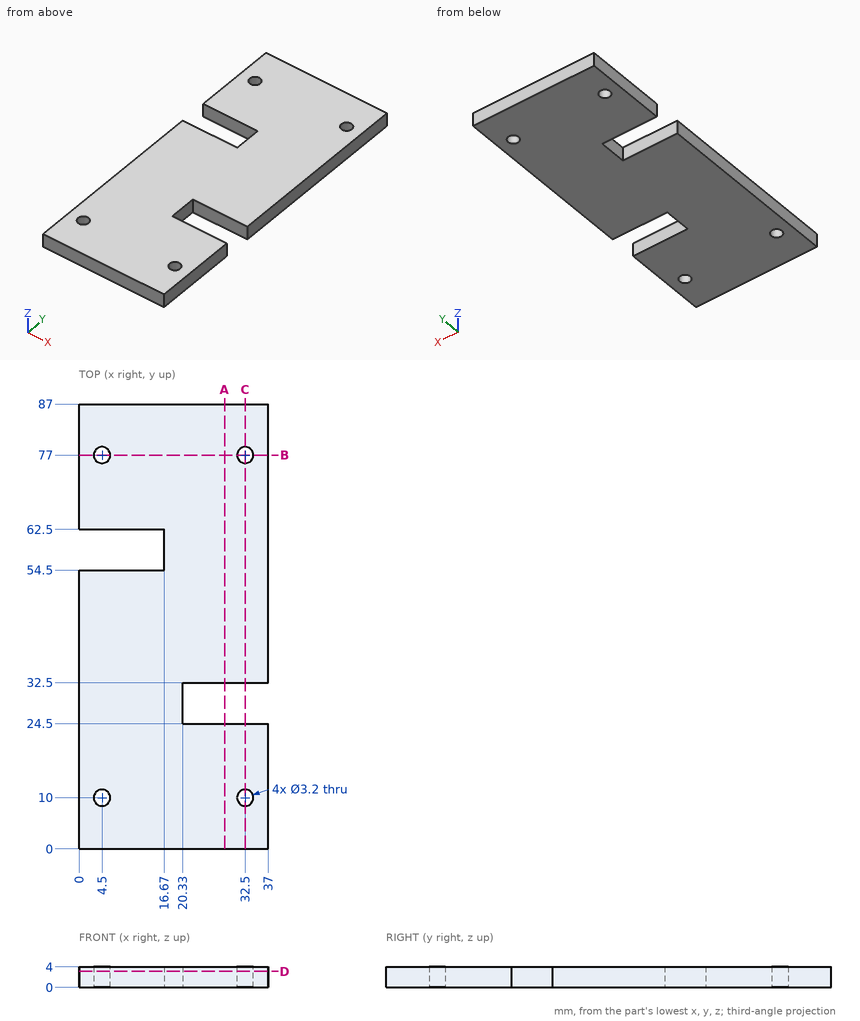
Geometry check sheet. Reference: drawing and pictorial views, mm from the part's lowest x, y, z. Give positions to 0.01 mm unless a question says otherwise; leave off trailing zeros. Order: outer loops, then holes, each group sorted by start corner. A loop starts at its lowest first (then second) coordinate and runs counter-clockwise, first axis right, second up. Notation, with made-up numbers: (58.5, -36) -> (87.5, -36) arc R31 cw to (87.5, -3) -> close; hole circle Ø4 at (22.5, 9). An arc over 180 degrees is marked (long way). Use CSV: the item, a comma, the result in double quotes. Start each with the question number.
1) Sectioned sample at D-D, the plane z = 3.1. Record the boundary of the cut face in (x, y).
2) Sectioned sample at A-A, the plane x = 28.5. Record the boundary of the cut face in (y, z).
3) Go/stop test with a flat-tipped pin: P1, Ø5, axis at x = 4.5, y = 77, coming from the -Z side. Record where the tip stops, or that it passes through.
4) Sectioned sample at B-B, the plane y = 77. Record the boundary of the cut face in (x, z), plus the area to 3 significant figures.
5) Sectioned sample at C-C, the plane x = 32.5. Record the boundary of the cut face in (y, z).
6) Material ranges on line 1 (Y direction, x = 4.5, z = 2.4); line 2 (X direction, y = 77, z = 2.7); line 3 (Y direction, x = 32.5, z = 3), recorded low to high. Write a range as from..to.
Recorded:
1,outline,"(0, 0) -> (37, 0) -> (37, 24.5) -> (20.33, 24.5) -> (20.33, 32.5) -> (37, 32.5) -> (37, 87) -> (0, 87) -> (0, 62.5) -> (16.67, 62.5) -> (16.67, 54.5) -> (0, 54.5) -> close; hole circle Ø3.2 at (4.5, 10); hole circle Ø3.2 at (4.5, 77); hole circle Ø3.2 at (32.5, 10); hole circle Ø3.2 at (32.5, 77)"
2,outline,"(0, 0) -> (24.5, 0) -> (24.5, 4) -> (0, 4) -> close; (32.5, 0) -> (87, 0) -> (87, 4) -> (32.5, 4) -> close"
3,P1,"z = 0"
4,outline,"(0, 0) -> (2.9, 0) -> (2.9, 4) -> (0, 4) -> close; (6.1, 0) -> (30.9, 0) -> (30.9, 4) -> (6.1, 4) -> close; (34.1, 0) -> (37, 0) -> (37, 4) -> (34.1, 4) -> close"
4,area,"122 mm2"
5,outline,"(0, 0) -> (8.4, 0) -> (8.4, 4) -> (0, 4) -> close; (11.6, 0) -> (24.5, 0) -> (24.5, 4) -> (11.6, 4) -> close; (32.5, 0) -> (75.4, 0) -> (75.4, 4) -> (32.5, 4) -> close; (78.6, 0) -> (87, 0) -> (87, 4) -> (78.6, 4) -> close"
6,line 1,"0..8.4, 11.6..54.5, 62.5..75.4, 78.6..87"
6,line 2,"0..2.9, 6.1..30.9, 34.1..37"
6,line 3,"0..8.4, 11.6..24.5, 32.5..75.4, 78.6..87"
